Could you check a few things on this model? Use its own coordinates, in mm. Face numbers are marked on the shaded views. A direction names the side the tool comes from. Give positions to 0.01 mm unless a question says otherwise; leave off trailing zeros. Order: outer loops, then holes, each group sorted by start corner. A loop starts at its lowest first (then second) coordinate and runs counter-clockwise, first axis right, second up. Notation, with made-up numbers: (-21, 4) - (2, 4) arc R24 cw to (2, 15) - close; hole circle Ø5 at (21.5, 83.5). An arc over 180 degrees is marked (long way). Put each result on its own line as item: value.
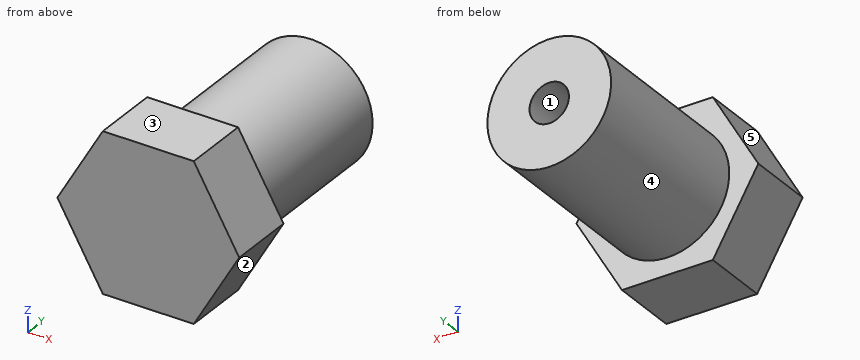
from build123d import *

# Parameters (mm, degrees)
BOSS_EXTRUDE1_DEPTH = 6
SKETCH2_R           = 5.5
SKETCH2_R_2         = 1.75
BOSS_EXTRUDE2_DEPTH = 16


with BuildPart() as part:
    # Sketch1 → Boss-Extrude1 (new body)
    with BuildSketch(Plane(origin=(0, 0, 0), x_dir=(1, 0, 0), z_dir=(0, 1, 0))):
        Polygon((8.082903769, 0), (4.041451884, 7), (-4.041451884, 7), (-8.082903769, 0), (-4.041451884, -7), (4.041451884, -7), align=None)
    extrude(amount=BOSS_EXTRUDE1_DEPTH)

    # Sketch2 → Boss-Extrude2 (add)
    with BuildSketch(Plane(origin=(0, 6, 0), x_dir=(1, 0, 0), z_dir=(0, 1, 0))):
        Circle(SKETCH2_R)
        Circle(SKETCH2_R_2, mode=Mode.SUBTRACT)
    extrude(amount=BOSS_EXTRUDE2_DEPTH)


solid = part.part
1) Suppose I cut it at C-C, the plane z = 1. List the corners of the cut face in (x, y) for me, and give its area (3 significant figures).
Filled in:
outline: (-7.51, 0) - (7.51, 0) - (7.51, 6) - (5.41, 6) - (5.41, 22) - (1.44, 22) - (1.44, 6) - (-1.44, 6) - (-1.44, 22) - (-5.41, 22) - (-5.41, 6) - (-7.51, 6) - close
area: 217 mm^2
2) I'm going to push flat-ended pins straight in: pin 1 (6 mm diameter, centred on x = -2, y = 17.5, fed in from -Z); pin 2 (3 mm diameter, centred on y = 9.5, z = -1, fed in from +X); pin 3 (1.8 mm diameter, centred on x = -0.5, z = 0, fed in from +Y). Where does each tip first touch, or does it pass through?
Filled in:
pin 1: stops at z = -5.5
pin 2: stops at x = 5.5
pin 3: stops at y = 6
3) If I drill on line 1 (Z direction, x = 0, y = 11.25); line 2 (Y direction, x = 3.75, z = -5.25), over which ranges is the centre line in solid material (lowest first)? Write a range as [from, to].
Filled in:
line 1: z = [-5.5, -1.75], [1.75, 5.5]
line 2: y = [0, 6]
4) Suppose I cut it at D-D, the plane y = 7.25. List the corners of the cut face in (x, z) for me.
Filled in:
outline: circle Ø11 at (0, 0); hole circle Ø3.5 at (0, 0)
5) Suppose I cut it at B-B, the plane y = 2.5. List the corners of the cut face in (x, z) for me, and give its area (3 significant figures).
Filled in:
outline: (-8.08, 0) - (-4.04, -7) - (4.04, -7) - (8.08, 0) - (4.04, 7) - (-4.04, 7) - close
area: 170 mm^2
6) Which directions (+Z, -Z, +X, -X, +Y, -Y) give clear straight access to the entire face, cutting with the end or side of a thin tool? Please do the marked faces 4 and 5.
Filled in:
face 4: +Y
face 5: +Z, -X, +Y, -Y
7) We'd pull the mould along Z, two halves only. Please class the marked faces 1, 2 and 3: pulls with the +Z half, pulls with the -Z half, needs draft (parallel to the pull), parting line crosses it, or undercut.
Filled in:
face 1: undercut
face 2: pulls with the -Z half
face 3: pulls with the +Z half
8) Suppose I cut it at A-A, the plane x = 0. List the corners of the cut face in (y, z) for me, and give its area (3 significant figures).
Filled in:
outline: (0, -7) - (6, -7) - (6, -5.5) - (22, -5.5) - (22, -1.75) - (6, -1.75) - (6, 1.75) - (22, 1.75) - (22, 5.5) - (6, 5.5) - (6, 7) - (0, 7) - close
area: 204 mm^2
